The model under review builds one solid part; all positions refer to its coordinate system, in mm. Face numbers are marked on the shaded views. A direction names the side the tool comes from. Give positions to 0.01 mm unless a question says otherwise; leave off trailing zeros. Loops run counter-clockwise (first coordinate to the right, second up) from the corner with the lowest first, then second, coordinate; pieces in that order, holes last. Notation, with made-up numbers: M 78.5,3.5 L 117.5,3.5 A21 ccw 117.5,33.5 Z; hole C 30.25,-3.5 d3. An arc over 180 degrees is marked long. Put each result on its own line as item: value. Start each with the question number.
from build123d import *

# Parameters (mm, degrees)
F0_R      = 50.8
F1_DEPTH  = 41.4476916194
F2_W      = 50.8
F2_H      = 50.8
F3_DEPTH  = 143.017962575
F4_R      = 12.7
F5_DEPTH  = 76.201
F6_R      = 5.08
F7_R      = 19.05
F8_DEPTH  = 184.4666541944
F9_R      = 25.4
F9_R_2    = 19.05
F10_DEPTH = 72.4607035518


with BuildPart() as f1:
    # F0 (on Top) → F1 (new body)
    with BuildSketch(Plane.XY):
        Circle(F0_R)
    extrude(amount=-F1_DEPTH)

    # F2 (on face) → F3 (join)
    with BuildSketch(Plane.XY):
        Rectangle(F2_W, F2_H)
    extrude(amount=F3_DEPTH)

    # F4 (on face) → F5 (cut, through all)
    with BuildSketch(Plane.YZ.offset(25.4)):
        with Locations((0, 101.6)):
            Circle(F4_R)
    extrude(amount=-F5_DEPTH, mode=Mode.SUBTRACT)

    # F6
    f6_edges = [f1.edges().sort_by_distance(p)[0] for p in [
        (25.4, 25.4, 71.508981),
        (-25.4, 25.4, 71.508981),
        (0, 25.4, 0),
        (0, 25.4, 143.017963),
        (25.4, -25.4, 71.508981),
        (25.4, 0, 0),
        (25.4, 0, 143.017963),
        (25.4, -12.7, 101.6),
        (-25.4, -25.4, 71.508981),
        (0, -25.4, 0),
        (0, -25.4, 143.017963),
        (-25.4, 0, 0),
    ]]
    fillet(f6_edges, radius=F6_R)

    # F7 (on face) → F8 (cut, through all)
    with BuildSketch(Plane(origin=(0, 0, -41.4476916194), x_dir=(1, 0, 0), z_dir=(0, 0, -1))):
        Circle(F7_R)
    extrude(amount=-F8_DEPTH, mode=Mode.SUBTRACT)

    # F9 (on face) → F10 (join)
    with BuildSketch(Plane(origin=(0, 0, -41.4476916194), x_dir=(1, 0, 0), z_dir=(0, 0, -1))):
        Circle(F9_R)
        Circle(F9_R_2, mode=Mode.SUBTRACT)
    extrude(amount=F10_DEPTH)


solid = f1.part
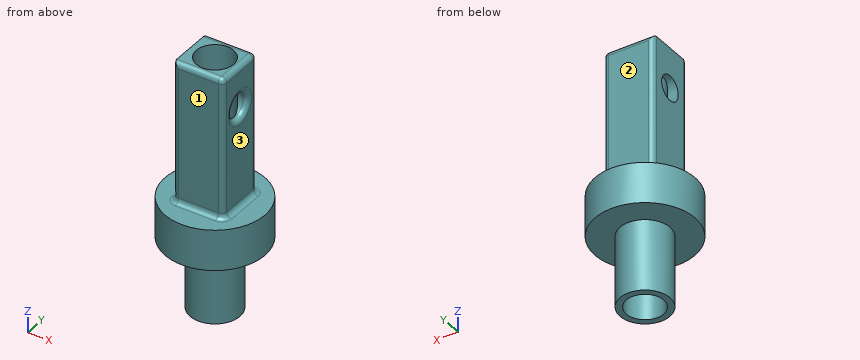
(1) To check wall thickness, follow L1, parallel to Y at x = 15.75, z = 101.6; L2, parallel to Z at x = -21, y = 0; L3, parallel to Y at x = 0, z = -57. State the ranges of each line that lie inside material, in increasing order. Write a range as [from, to].
(2) For the marked faces 1, 2 and 3, list the 3-axis set-ups (+Z, -Z, +X, -X, +Y, -Y) from which the entire face can be reached by the end or side of a thin tool; tool diameter is ignored.
(3) We need section A-A, the plane x = 0. Write out the cut boundary in (y, z), plus the area to 3 significant figures.
(4) We need section B-B, the plane z = 101.6. Write out the cut boundary in (x, y), plus the area to 3 significant figures.
(5) Insertion check: pin 1 (1 mm diameter, centred on x = 35.5, z = -37.5, fed in from +Y); pin 2 (1.5 mm diameter, centred on x = 30, z = -28, fed in from +Y); pin 3 (5 mm diameter, centred on y = 7, z = -59, fed in from -X). Each pin has a flat end and moves straight along its axis. Give the tip position at first contact, or say it passes through.
(6) We need section C-C, the plane z = 70.5. Write out the cut boundary in (x, y).
(7) We need section D-D, the plane y = 0. State how many separate pieces and enclosed holes the cut face has, plus the area to 3 significant figures.
Check sheet entries:
1. L1: y = [-25.4, -12.7], [12.7, 25.4]
1. L2: z = [-113.91, 88.9], [114.3, 143.02]
1. L3: y = [-25.4, -19.05], [19.05, 25.4]
2. face 1: +Z, +X, -X, -Y
2. face 2: +Z, +X, -X, +Y
2. face 3: +Z, +X, +Y, -Y
3. outline: M -50.8,-41.45 L -25.4,-41.45 L -25.4,-113.91 L -19.05,-113.91 L -19.05,143.02 L -20.32,143.02 A5.08 ccw -25.4,137.94 L -25.4,5.08 A5.08 cw -30.48,0 L -50.8,0 Z; M 19.05,-113.91 L 25.4,-113.91 L 25.4,-41.45 L 50.8,-41.45 L 50.8,0 L 30.48,0 A5.08 cw 25.4,5.08 L 25.4,137.94 A5.08 ccw 20.32,143.02 L 19.05,143.02 Z
3. area: 5,370 mm²
4. outline: M -25.4,-20.32 A5.08 ccw -20.32,-25.4 L 20.32,-25.4 A5.08 ccw 25.4,-20.32 L 25.4,-17.78 A5.08 ccw 20.32,-12.7 L 14.2,-12.7 A19.05 cw -14.2,-12.7 L -25.4,-12.7 Z; M -25.4,12.7 L -14.2,12.7 A19.05 cw 14.2,12.7 L 20.32,12.7 A5.08 ccw 25.4,17.78 L 25.4,20.32 A5.08 ccw 20.32,25.4 L -20.32,25.4 A5.08 ccw -25.4,20.32 Z
4. area: 1,010 mm²
5. pin 1: stops at y = 36.82
5. pin 2: stops at y = 41.53
5. pin 3: stops at x = -25
6. outline: M -25.4,-20.32 A5.08 ccw -20.32,-25.4 L 20.32,-25.4 A5.08 ccw 25.4,-20.32 L 25.4,20.32 A5.08 ccw 20.32,25.4 L -20.32,25.4 A5.08 ccw -25.4,20.32 Z; hole C 0,0 d38.1
7. separate pieces: 4
7. enclosed holes: 0
7. area: 5,040 mm²
